from build123d import *

# Parameters (mm, degrees)
SKETCH1_W                = 40
SKETCH1_H                = 56
BOSS_EXTRUDE1_DEPTH      = 14
SKETCH5_W                = 13
SKETCH5_H                = 7
CUT_EXTRUDE1_DEPTH       = 68
SKETCH7_R                = 7
BOSS_EXTRUDE2_DEPTH      = 14
BOSS_EXTRUDE3_DEPTH      = 8
BOSS_EXTRUDE3_DEPTH_BACK = 1
SKETCH8_R                = 11
SKETCH9_R                = 6
CUT_EXTRUDE2_DEPTH       = 44


with BuildPart() as part:
    # Sketch1 → Boss-Extrude1 (new body)
    with BuildSketch(Plane(origin=(0, 0, 0), x_dir=(1, 0, 0), z_dir=(0, 1, 0))):
        with Locations((0, -28)):
            Rectangle(SKETCH1_W, SKETCH1_H)
    extrude(amount=BOSS_EXTRUDE1_DEPTH)

    # Sketch5 → Cut-Extrude1 (cut)
    with BuildSketch(Plane.XY):
        with Locations((6.5, 3.5)):
            Rectangle(SKETCH5_W, SKETCH5_H)
        with Locations((-6.5, 3.5)):
            Rectangle(SKETCH5_W, SKETCH5_H)
    extrude(amount=CUT_EXTRUDE1_DEPTH, mode=Mode.SUBTRACT)

    # Sketch7 → Boss-Extrude2 (add)
    with BuildSketch(Plane.XY):
        with BuildLine():
            Line((20, 14), (-20, 14))
            Line((-20, 14), (-11.528805322, 43.329811826))
            ThreePointArc((-11.528805322, 43.329811826), (0, 52.000041623), (11.528805322, 43.329811826))
            Line((11.528805322, 43.329811826), (20, 14))
        make_face()
        with Locations((0, 40)):
            Circle(SKETCH7_R, mode=Mode.SUBTRACT)
    extrude(amount=BOSS_EXTRUDE2_DEPTH)

    # Sketch8 → Boss-Extrude3 (add, two sides: drawn at the far end of the back side and taken through both)
    with BuildSketch(Plane(origin=(0, 14, 0), x_dir=(1, 0, 0), z_dir=(0, 1, 0)).offset(-BOSS_EXTRUDE3_DEPTH_BACK)):
        with Locations(Location((0, -36, 0), (0, 0, 270))):
            Circle(SKETCH8_R)
    extrude(amount=BOSS_EXTRUDE3_DEPTH + BOSS_EXTRUDE3_DEPTH_BACK)

    # Sketch9 → Cut-Extrude2 (cut)
    with BuildSketch(Plane(origin=(0, 22, 0), x_dir=(1, 0, 0), z_dir=(0, 1, 0))):
        with Locations(Location((0, -36, 0), (0, 0, 270))):
            Circle(SKETCH9_R)
    extrude(amount=-CUT_EXTRUDE2_DEPTH, mode=Mode.SUBTRACT)


solid = part.part
For this review, take the finished solid that the model builds, in its own axes (mm). A direction names the side the tool comes from. Round coordinates to 2 decimals unless told otherwise and drop trailing zeros. Order: outer loops, then holes, each group sorted by start corner. A loop starts at its lowest first (then second) coordinate and runs counter-clockwise, first axis right, second up. Notation, with made-up numbers: (-7, -2.75) -> (0, -2.75) arc R12 cw to (0, 3.25) -> close; hole circle Ø1 at (22.5, -9.5). An arc over 180 degrees is marked (long way). Put each result on its own line as item: value.
Q1. Machinability: for faces 5 (the flat face through (-5, 22, 41)), 6 (the flat face through (-5, 14, 25)), 7 (the flat face through (0, 29, 14)), 8 (the flat face through (13, 3, 28)), which of the approach directions +Z, -Z, +X, -X, +Y, -Y give a long, thin tool a straight path to every point of the face, cutting with its end or side? Answer none if there is none.
Check result:
face 5: +Z, +X, -X, +Y
face 6: +Y
face 7: +X, -X, +Y
face 8: +Z, -Z, -Y
Q2. Add section C-C on y = 40. Write out the cut boundary in (x, z), plus the area to 3 significant figures.
Check result:
outline: (-12.49, 0) -> (-7, 0) -> (-7, 14) -> (-12.49, 14) -> close; (7, 0) -> (12.49, 0) -> (12.49, 14) -> (7, 14) -> close
area: 154 mm2
Q3. Add section D-D on z = 49. Write out the cut boundary in (x, y).
Check result:
outline: (-20, 0) -> (-13, 0) -> (-13, 7) -> (13, 7) -> (13, 0) -> (20, 0) -> (20, 14) -> (-20, 14) -> close
Q4. Mouldability with a two-part tool opening along X and no side actions: class faces 1 (the flat face through (20, 7, 28)), 2 (the cylindrical face through (-0.91, 46.94, 6.9)), 3 (the flat face through (0, 7, 28)), 4 (the flat face through (-15.824, 28.46, 6.902)) as pulls with the +X half, pulls with the -X half, needs draft (parallel to the pull), parting line crosses it, or undercut.
Check result:
face 1: pulls with the +X half
face 2: undercut
face 3: undercut
face 4: pulls with the -X half
Q5. For probe 1 along X at (y, z) = (4, 20); probe 2 along X at (y, z) = (16, 36); probe 3 along Z at (x, y) = (13.5, 22.5), list the stretches that pass through material, from the lowest coordinate up. Write a range as [from, to].
Check result:
probe 1: [-20, -13], [13, 20]
probe 2: [-11, -6], [6, 11]
probe 3: [0, 14]
Q6. Add section A-A on x = 0. Write out the cut boundary in (y, z).
Check result:
outline: (7, 0) -> (33, 0) -> (33, 14) -> (14, 14) -> (14, 25) -> (22, 25) -> (22, 30) -> (7, 30) -> close; (7, 42) -> (22, 42) -> (22, 47) -> (14, 47) -> (14, 56) -> (7, 56) -> close; (47, 0) -> (52, 0) -> (52, 14) -> (47, 14) -> close
Q7. Add section B-B on z = 36. Write out the cut boundary in (x, y), plus the area to 3 significant figures.
Check result:
outline: (-20, 0) -> (-13, 0) -> (-13, 7) -> (-6, 7) -> (-6, 22) -> (-11, 22) -> (-11, 14) -> (-20, 14) -> close; (6, 7) -> (13, 7) -> (13, 0) -> (20, 0) -> (20, 14) -> (11, 14) -> (11, 22) -> (6, 22) -> close
area: 374 mm2
Q8. Insertion check: pin 1 Ø2 at (x, z) = (-8.5, 16.5) entering from -Y; pin 2 Ø1 at (x, y) = (1.5, 29) entering from +Z; pin 3 Ø1.5 at (x, y) = (-8, 5) entering from -Z; pin 4 Ø12 at (x, z) = (6.5, 33) entering from +Y. Each pin has a flat end and moves straight along its axis. Give the tip position at first contact, or say it passes through.
Check result:
pin 1: y = 7
pin 2: z = 14
pin 3: through
pin 4: y = 22
